For this review, take the finished solid that the model builds, in its own axes (mm). A direction names the side the tool comes from. Round coordinates to 2 decimals unless told otherwise and drop trailing zeros. Write each loop counter-clockwise with the first axis right and the second up, starting at its lowest first coordinate (ties: lowest second). Pieces come first, ordered by that corner, then holes. Notation, with made-up numbers: (27.5, 6) -> (86.5, 6) arc R22 ccw to (86.5, 42) -> close; hole circle Ø1 at (52, 43.5). An arc over 180 degrees is marked (long way). Write item = value, one per line. Start each with the question number.
```python
from build123d import *

# Parameters (mm, degrees)
F0_R          = 3
F0_R_2        = 2.5
F1_DEPTH      = 621.5
F2_R          = 2
F3_R          = 7
F6_DEPTH      = 30
F6_DEPTH_BACK = 30


# Not quite as in the source:
# - a feature names something its author has since deleted; it is built from what else it names


with BuildPart() as f1:
    # F0 (on Top) → F1 (new body)
    with BuildSketch(Plane.XY):
        with BuildLine():
            Line((18.15, -30), (30, -30))
            Line((30, -30), (30, -18.15))
            Line((30, -18.15), (27.5, -18.15))
            Line((27.5, -18.15), (27.5, -20.15))
            Line((27.5, -20.15), (21.5477069044, -20.15))
            ThreePointArc((21.5477069044, -20.15), (19.5, -15), (21.5477069044, -9.85))
            Line((21.5477069044, -9.85), (27.5, -9.85))
            Line((27.5, -9.85), (27.5, -11.85))
            Line((27.5, -11.85), (30, -11.85))
            Line((30, -11.85), (30, 11.85))
            Line((30, 11.85), (27.5, 11.85))
            Line((27.5, 11.85), (27.5, 9.85))
            Line((27.5, 9.85), (21.5477069044, 9.85))
            ThreePointArc((21.5477069044, 9.85), (19.5, 15), (21.5477069044, 20.15))
            Line((21.5477069044, 20.15), (27.5, 20.15))
            Line((27.5, 20.15), (27.5, 18.15))
            Line((27.5, 18.15), (30, 18.15))
            Line((30, 18.15), (30, 30))
            Line((30, 30), (18.15, 30))
            Line((18.15, 30), (18.15, 27.5))
            Line((18.15, 27.5), (20.15, 27.5))
            Line((20.15, 27.5), (20.15, 21.5477069044))
            ThreePointArc((20.15, 21.5477069044), (15, 19.5), (9.85, 21.5477069044))
            Line((9.85, 21.5477069044), (9.85, 27.5))
            Line((9.85, 27.5), (11.85, 27.5))
            Line((11.85, 27.5), (11.85, 30))
            Line((11.85, 30), (-11.85, 30))
            Line((-11.85, 30), (-11.85, 27.5))
            Line((-11.85, 27.5), (-9.85, 27.5))
            Line((-9.85, 27.5), (-9.85, 21.5477069044))
            ThreePointArc((-9.85, 21.5477069044), (-15, 19.5), (-20.15, 21.5477069044))
            Line((-20.15, 21.5477069044), (-20.15, 27.5))
            Line((-20.15, 27.5), (-18.15, 27.5))
            Line((-18.15, 27.5), (-18.15, 30))
            Line((-18.15, 30), (-30, 30))
            Line((-30, 30), (-30, 18.15))
            Line((-30, 18.15), (-27.5, 18.15))
            Line((-27.5, 18.15), (-27.5, 20.15))
            Line((-27.5, 20.15), (-21.5477069044, 20.15))
            ThreePointArc((-21.5477069044, 20.15), (-19.5, 15), (-21.5477069044, 9.85))
            Line((-21.5477069044, 9.85), (-27.5, 9.85))
            Line((-27.5, 9.85), (-27.5, 11.85))
            Line((-27.5, 11.85), (-30, 11.85))
            Line((-30, 11.85), (-30, -11.85))
            Line((-30, -11.85), (-27.5, -11.85))
            Line((-27.5, -11.85), (-27.5, -9.85))
            Line((-27.5, -9.85), (-21.5477069044, -9.85))
            ThreePointArc((-21.5477069044, -9.85), (-19.5, -15), (-21.5477069044, -20.15))
            Line((-21.5477069044, -20.15), (-27.5, -20.15))
            Line((-27.5, -20.15), (-27.5, -18.15))
            Line((-27.5, -18.15), (-30, -18.15))
            Line((-30, -18.15), (-30, -30))
            Line((-30, -30), (-18.15, -30))
            Line((-18.15, -30), (-18.15, -27.5))
            Line((-18.15, -27.5), (-20.15, -27.5))
            Line((-20.15, -27.5), (-20.15, -21.5477069044))
            ThreePointArc((-20.15, -21.5477069044), (-15, -19.5), (-9.85, -21.5477069044))
            Line((-9.85, -21.5477069044), (-9.85, -27.5))
            Line((-9.85, -27.5), (-11.85, -27.5))
            Line((-11.85, -27.5), (-11.85, -30))
            Line((-11.85, -30), (11.85, -30))
            Line((11.85, -30), (11.85, -27.5))
            Line((11.85, -27.5), (9.85, -27.5))
            Line((9.85, -27.5), (9.85, -21.5477069044))
            ThreePointArc((9.85, -21.5477069044), (15, -19.5), (20.15, -21.5477069044))
            Line((20.15, -21.5477069044), (20.15, -27.5))
            Line((20.15, -27.5), (18.15, -27.5))
            Line((18.15, -27.5), (18.15, -30))
        make_face()
        with Locations((-25, -25)):
            Circle(F0_R, mode=Mode.SUBTRACT)
        with Locations((-15, -15)):
            Circle(F0_R_2, mode=Mode.SUBTRACT)
        with Locations((25, -25)):
            Circle(F0_R, mode=Mode.SUBTRACT)
        with Locations((15, -15)):
            Circle(F0_R_2, mode=Mode.SUBTRACT)
        with Locations((-25, 25)):
            Circle(F0_R, mode=Mode.SUBTRACT)
        with Locations((-15, 15)):
            Circle(F0_R_2, mode=Mode.SUBTRACT)
        Polygon((-7, 22), (-7, 27.5), (0, 27.5), (7, 27.5), (7, 22), (10, 16), (10, 10), (16, 10), (22, 7), (27.5, 7), (27.5, 0), (27.5, -7), (22, -7), (16, -10), (10, -10), (10, -16), (7, -22), (7, -27.5), (0, -27.5), (-7, -27.5), (-7, -22), (-10, -16), (-10, -10), (-16, -10), (-22, -7), (-27.5, -7), (-27.5, 0), (-27.5, 7), (-22, 7), (-16, 10), (-10, 10), (-10, 16), align=None, mode=Mode.SUBTRACT)
        with Locations((15, 15)):
            Circle(F0_R_2, mode=Mode.SUBTRACT)
        with Locations((25, 25)):
            Circle(F0_R, mode=Mode.SUBTRACT)
    extrude(amount=F1_DEPTH)

    # F2
    f2_edges = [f1.edges().sort_by_distance(p)[0] for p in [
        (-7, 27.5, 310.75),
        (7, 27.5, 310.75),
    ]]
    fillet(f2_edges, radius=F2_R)

    # F3
    f3_edges = [f1.edges().sort_by_distance(p)[0] for p in [
        (-10, 16, 310.75),
        (10, 16, 310.75),
    ]]
    fillet(f3_edges, radius=F3_R)

    # F5 (on Front) → F6 (cut, two sides)
    with BuildSketch(Plane.XZ) as f6_sk:
        Polygon((30, 621.5), (-11.184961555, 720.929292752), (-183.3312368923, 649.6239707953), (-142.1462753372, 550.1946780433), align=None)
    extrude(amount=F6_DEPTH, mode=Mode.SUBTRACT)
    extrude(f6_sk.sketch, amount=-F6_DEPTH_BACK, mode=Mode.SUBTRACT)


solid = f1.part
```
1. Wall thickness on L1, parallel to X at y = 25, z = 313.5; L2, parallel to Y at x = 15, z = 236: over which ranges is each line inside the solid? List them lowest first. Write a range as from..to.
2. Consider section A-A, the plane y = -1.5. Give the boundary of the cut face in (x, z), then the cut area to 3 significant figures.
3. Machinability: for faces 4 (the flat face through (0, -30, 303)), 5 (the cylindrical face through (19.5, 14.9, 304.7)), which of the approach directions +Z, -Z, +X, -X, +Y, -Y give a long, thin tool a straight path to every point of the face, cutting with its end or side? Answer none if there is none.
4. Draft analysis for pull direction X (two halves, no side actions). For faces 1 (the flat face through (-30, -24, 294)), 2 (the flat face through (30, 24, 306)), 3 (the flat face through (27.5, 0, 306)), state which applies: +X half, -X half, draft (parallel to the pull), parting line (faces both ways), or undercut.
5. Clearance check with flat-ended pins moving along their axes: pin 1 Ø1.8 at (y, z) = (-14, 297.5) entering from -X; pin 2 Ø4 at (x, y) = (18.5, -23) entering from +Z (3 decimals). State where each tip first meets the part, or that it passes through.
6. Consider section B-B, the plane z = 348. Give the number of separate pieces and of enclosed holes in the cut face, then the cut area to 3 significant figures.
Outcome:
q1.L1 = -30..-28, -22..-20.15, -9.85..-7, 7..9.85, 20.15..22, 28..30
q1.L2 = -19.5..-17.5, -12.5..-10, 10..12.5, 17.5..19.5
q2.outline = (-30, 0) -> (-27.5, 0) -> (-27.5, 597.68) -> (-30, 596.65) -> close; (27.5, 0) -> (30, 0) -> (30, 621.5) -> (27.5, 620.46) -> close
q2.area = 3,050 mm2
q3.face_4 = +Z, -Z, +X, -X, -Y
q3.face_5 = +Z, -Z
q4.face_1 = -X half
q4.face_2 = +X half
q4.face_3 = undercut
q5.pin_1 = -19.74
q5.pin_2 = 617.565
q6.separate_pieces = 1
q6.enclosed_holes = 9
q6.area = 1,080 mm2
